```python
from build123d import *

# Parameters (mm, degrees)
F1_DEPTH  = 21
F2_R      = 2
F3_DEPTH  = 50
F4_R      = 4.5
F5_DEPTH  = 4
F6_R      = 4.5
F7_DEPTH  = 4
F8_R      = 2
F9_DEPTH  = 15
F11_DEPTH = 12


with BuildPart() as f1:
    # F0 (on Front) → F1 (new body)
    with BuildSketch(Plane.XZ):
        with BuildLine():
            ThreePointArc((44.619485, -22.56328), (39.527789, -30.619502), (33, -37.56328))
            Line((33, -37.56328), (33, -79))
            Line((33, -79), (18.995849, -99))
            Line((18.995849, -99), (0, -99))
            Line((0, -99), (-33, -99))
            Line((-33, -99), (-33, -37.56328))
            ThreePointArc((-33, -37.56328), (-39.527789, -30.619502), (-44.619485, -22.56328))
            Line((-44.619485, -22.56328), (-50, -22.56328))
            Line((-50, -22.56328), (-50, -133))
            Line((-50, -133), (-33, -150))
            Line((-33, -150), (-33, -180))
            Line((-33, -180), (-33, -197))
            Line((-33, -197), (0, -197))
            Line((0, -197), (33, -197))
            Line((33, -197), (33, -180))
            Line((33, -180), (33, -150))
            Line((33, -150), (50, -133))
            Line((50, -133), (50, -22.56328))
            Line((50, -22.56328), (44.619485, -22.56328))
        make_face()
    extrude(amount=F1_DEPTH)

    # F2 (on Right) → F3 (cut, symmetric)
    with BuildSketch(Plane.YZ):
        with Locations((-10.5, -55.10355)):
            Circle(F2_R)
        with Locations((-10.5, -85.60355)):
            Circle(F2_R)
    extrude(amount=F3_DEPTH, both=True, mode=Mode.SUBTRACT)

    # F4 (on face) → F5 (cut)
    with BuildSketch(Plane(origin=(-50, 0, 0), x_dir=(0, -1, 0), z_dir=(-1, 0, 0))):
        with Locations((10.5, -55.10355)):
            Circle(F4_R)
        with Locations((10.5, -85.60355)):
            Circle(F4_R)
    extrude(amount=-F5_DEPTH, mode=Mode.SUBTRACT)

    # F6 (on face) → F7 (cut)
    with BuildSketch(Plane.YZ.offset(50)):
        with Locations((-10.5, -55.10355)):
            Circle(F6_R)
        with Locations((-10.5, -85.60355)):
            Circle(F6_R)
    extrude(amount=-F7_DEPTH, mode=Mode.SUBTRACT)

    # F8 (on face) → F9 (cut)
    with BuildSketch(Plane(origin=(0, 0, -197), x_dir=(1, 0, 0), z_dir=(0, 0, -1))):
        with BuildLine():
            ThreePointArc((-23, 10.5), (-21, 8.5), (-19, 10.5))
            ThreePointArc((-19, 10.5), (-21, 12.5), (-23, 10.5))
        make_face()
        with Locations((21, 10.5)):
            Circle(F8_R)
    extrude(amount=-F9_DEPTH, mode=Mode.SUBTRACT)

    # F10 (on face) → F11 (cut)
    with BuildSketch(Plane.XZ.offset(21)):
        with BuildLine():
            ThreePointArc((0, -166.5), (-2, -168.5), (0, -170.5))
            Line((0, -170.5), (0, -166.5))
        make_face()
        with BuildLine():
            ThreePointArc((0, -131), (-2, -133), (0, -135))
            Line((0, -135), (0, -131))
        make_face()
        with BuildLine():
            Line((0, -131), (0, -135))
            ThreePointArc((0, -135), (1.414214, -134.414214), (2, -133))
            ThreePointArc((2, -133), (1.414214, -131.585786), (0, -131))
        make_face()
        with BuildLine():
            Line((0, -166.5), (0, -170.5))
            ThreePointArc((0, -170.5), (1.414214, -169.914214), (2, -168.5))
            ThreePointArc((2, -168.5), (1.414214, -167.085786), (0, -166.5))
        make_face()
    extrude(amount=-F11_DEPTH, mode=Mode.SUBTRACT)


solid = f1.part
```
Input: part model. Units: mm. Frame: model coordinates. A direction names the side the tool comes from. Coordinates: 2 decimals unless noted, no trailing zeros. Loops run counter-clockwise (first coordinate to the right, second up) from the corner with the lowest first, then second, coordinate; pieces in that order, holes last. Notation, with made-up numbers: M 45,29 L 62,29 A19 ccw 62,54 Z; hole C 58.25,-35 d6. An arc over 180 degrees is marked long. Use a Markdown table: item, result. Add a question column.
1) Set-up query: faces 4 (the flat face through (-46, -11, -88)), 5 (the cylindrical face through (48.03, -8.08, -51.31)), 6 (the flat face through (0, -9, -168)), 7 (the flat face through (-21, -11, -182)), 8 (the flat face through (26, -10, -89)). Return all of +Z, -Z, +X, -X, +Y, -Y with unobstructed straight access to the full face (end or side cutting, diameter ignored); none if empty.
2) Line query: L1, parallel to Y at x = -21, z = -187; L2, parallel to Z at x = 38.5, y = -10.5; L3, parallel to Z at x = 47.5, y = -10.5. Output: solid intervals per line, ascending. Write a range as from..to.
3) Section C-C, the plane x = 21. Return the cut outline in (y, z).
4) Draft query along X for faces 1 (the cylindrical face through (39.61, -10.35, -30.51)), 2 (the cylindrical face through (36.605, -10.934, -87.556)), 3 (the flat face through (-42, -10, -141)). Return one class per face: +X half, -X half, draft (parallel to the pull), parting line (faces both ways), or undercut.
5) Section A-A, the plane z = -72. Return the cut outline in (x, y).
6) Pin query (flat end, axial travel): P1, Ø2, axis at y = -3.5, z = -141, coming from the +X side; P2, Ø8, axis at x = -2, y = -11, coming from the +Z side; P3, Ø8, axis at y = -10.5, z = -85.6, coming from the -X side; P4, Ø2.5, axis at y = -10.5, z = -55.1, coming from the +X side. Return the tip coordinate at first contact, or that it passes through.
7) Section B-B, the plane y = -18.5. Return the cut outline in (x, z), plus the area to 3 significant figures.
8) Section D-D, the plane y = -2.5. Return the cut outline in (x, z), plus the area to 3 significant figures.
Answer below:
| question | item | result |
|---|---|---|
| 1 | face 4 | -X |
| 1 | face 5 | +X |
| 1 | face 6 | -Y |
| 1 | face 7 | -Z |
| 1 | face 8 | +Z, +Y, -Y |
| 2 | L1 | -21..-12.5, -8.5..0 |
| 2 | L2 | -144.5..-87.6, -83.6..-57.1, -53.1..-31.9 |
| 2 | L3 | -135.5..-90.1, -81.1..-59.6, -50.6..-22.56 |
| 3 | outline | M -21,-197 L -12.5,-197 L -12.5,-182 L -8.5,-182 L -8.5,-197 L 0,-197 L 0,-96.14 L -21,-96.14 Z |
| 4 | face 1 | undercut |
| 4 | face 2 | draft |
| 4 | face 3 | -X half |
| 5 | outline | M -50,-21 L -33,-21 L -33,0 L -50,0 Z; M 33,-21 L 50,-21 L 50,0 L 33,0 Z |
| 6 | P1 | x = 43 |
| 6 | P2 | z = -99 |
| 6 | P3 | x = -46 |
| 6 | P4 | through |
| 7 | outline | M -50,-133 L -33,-150 L -33,-197 L 33,-197 L 33,-150 L 50,-133 L 50,-22.56 L 44.62,-22.56 A50 cw 33,-37.56 L 33,-79 L 19,-99 L -33,-99 L -33,-37.56 A50 cw -44.62,-22.56 L -50,-22.56 Z; hole M 0,-170.5 A2 ccw 2,-168.5 A2 ccw 0,-166.5 A2 ccw Z; hole M 0,-135 A2 ccw 2,-133 A2 ccw 0,-131 A2 ccw Z |
| 7 | area | 10,400 mm2 |
| 8 | outline | M -50,-133 L -33,-150 L -33,-197 L 33,-197 L 33,-150 L 50,-133 L 50,-22.56 L 44.62,-22.56 A50 cw 33,-37.56 L 33,-79 L 19,-99 L -33,-99 L -33,-37.56 A50 cw -44.62,-22.56 L -50,-22.56 Z |
| 8 | area | 10,500 mm2 |
